```python
from build123d import *

# Parameters (mm, degrees)
CROQUIS4_R            = 95.5
CROQUIS4_R_2          = 79
CORTAR_EXTRUIR1_START = -79
CROQUIS6_R            = 85
CROQUIS6_R_2          = 79
CORTAR_EXTRUIR1_DEPTH = 79
CROQUIS7_R            = 85
CROQUIS7_R_2          = 79
CORTAR_EXTRUIR2_DEPTH = 79


with BuildPart() as part:
    # Barrer5: sweep along a path in Croquis3
    with BuildLine(Plane.XY) as barrer5_path:
        Line((0, 0), (0, 79))
        ThreePointArc((0, 79), (29.435768491, 150.064231509), (100.5, 179.5))
        Line((100.5, 179.5), (179.5, 179.5))
    # Croquis4 → Barrer5 (sweep)
    with BuildSketch(Plane(origin=(0, 0, 0), x_dir=(1, 0, 0), z_dir=(0, 1, 0))):
        Circle(CROQUIS4_R)
        Circle(CROQUIS4_R_2, mode=Mode.SUBTRACT)
    sweep(path=barrer5_path.line)

    # Croquis6 → Cortar-Extruir1 (cut)
    with BuildSketch(Plane.XZ.offset(CORTAR_EXTRUIR1_START)):
        with Locations(Location((0, 0, 0), (0, 0, 270))):
            Circle(CROQUIS6_R)
        Circle(CROQUIS6_R_2, mode=Mode.SUBTRACT)
    extrude(amount=CORTAR_EXTRUIR1_DEPTH, mode=Mode.SUBTRACT)

    # Croquis7 → Cortar-Extruir2 (cut)
    with BuildSketch(Plane(origin=(179.5, 0, 0), x_dir=(0, 0, -1), z_dir=(1, 0, 0))):
        with Locations(Location((0, 179.5, 0), (0, 0, 90))):
            Circle(CROQUIS7_R)
        with Locations((0, 179.5)):
            Circle(CROQUIS7_R_2, mode=Mode.SUBTRACT)
    extrude(amount=-CORTAR_EXTRUIR2_DEPTH, mode=Mode.SUBTRACT)


solid = part.part
```
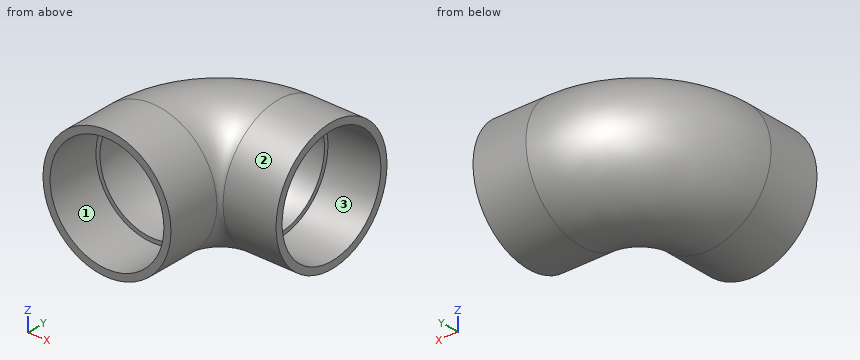
Read the model definition and answer for the solid it produces. Units are mm, in the model's axes. Face numbers are marked on the shaded views. Round coordinates to 2 decimals unless told otherwise and drop trailing zeros. Write each loop counter-clockwise with the first axis right and the second up, starting at its lowest first coordinate (ties: lowest second). Pieces come first, ordered by that corner, then holes. Notation, with made-up numbers: (82.5, 71.25) - (120.5, 71.25) arc R14 ccw to (120.5, 92.25) - close; hole circle Ø9 at (22.25, 2.25). An arc over 180 degrees is marked (long way). Use CSV: the item, a comma, the result in double quotes.
Q1. Find section B-B, the plane y = 73.5. Write down the section's boundary in (x, z), then the cut area to 3 significant figures.
Values:
outline,"circle Ø191 at (0, 0); hole circle Ø170 at (0, 0)"
area,"5,950 mm²"
Q2. Each of these flat-tipped pins is pushed along its axis until it touches: pin 1 Ø2 at (x, z) = (23, 47.5) entering from -Y; pin 2 Ø3 at (x, y) = (35, 240) entering from -Z; pin 3 Ø2 at (x, y) = (-61.5, 138) entering from -Z. Where does it stop, or does it pass through?
Values:
pin 1,"stops at y = 222.09"
pin 2,"stops at z = -62.95"
pin 3,"stops at z = -63.97"
Q3. Determine the mould class of the marked faces 1, 2 and 3 for opening direction Y: +Y half, -Y half, draft (parallel to the pull), parting line (faces both ways), or undercut.
Values:
face 1,"draft"
face 2,"parting line"
face 3,"undercut"
Q4. Straight lines are drawn through the part: line 1 along Z through (x, y) = (133, 179); line 2 along X through (y, z) = (47.5, -30). For each, find the intervals that lie inside material, in ascending order.
Values:
line 1,"z = -95.5 to -85, 85 to 95.5"
line 2,"x = -90.67 to -79.53, 79.53 to 90.67"
Q5. Find section A-A, the plane z = 0. Write down the section's boundary in (x, y).
Values:
outline,"(-95.5, 0) - (-85, 0) - (-85, 79) - (-79, 79) arc R179.5 cw to (100.5, 258.5) - (100.5, 264.5) - (179.5, 264.5) - (179.5, 275) - (100.5, 275) arc R196 ccw to (-95.5, 79) - close; (79, 79) - (85, 79) - (85, 0) - (95.5, 0) - (95.5, 79) arc R5 cw to (100.5, 84) - (179.5, 84) - (179.5, 94.5) - (100.5, 94.5) - (100.5, 100.5) arc R21.5 ccw to start"
Q6. Find section C-C, the plane z = -66. Write down the section's boundary in (x, y), then the cut area to 3 significant figures.
Values:
outline,"(-69.02, 0) - (-53.56, 0) - (-53.56, 79) - (-43.42, 79) arc R143.92 cw to (100.5, 222.92) - (100.5, 233.06) - (179.5, 233.06) - (179.5, 248.52) - (100.5, 248.52) arc R169.52 ccw to (-69.02, 79) - close; (43.42, 79) - (53.56, 79) - (53.56, 0) - (69.02, 0) - (69.02, 79) arc R31.48 cw to (100.5, 110.48) - (179.5, 110.48) - (179.5, 125.94) - (100.5, 125.94) - (100.5, 136.08) arc R57.08 ccw to start"
area,"13,000 mm²"
